Solid Edge part; units mm, degrees
sketch "Sketch1" plane through (0, 0, 0) normal (0, -1, 0) x (1, 0, 0)
  line L0 (-11.4484, 120) -> (-32.1539, 120)
  line L1 (-32.1539, 120) -> (0, 0)
  line L2 (0, 0) -> (20.7055, 0)
  line L3 (20.7055, 0) -> (-11.4484, 120)
extrude "Protrusion1" add sketch "Sketch1" against normal blind 20
hole "Agujero_3" at (-22.1539, 10, 120) direction (0, 0, -1) diameter 4.917 depth 24 tip angle 118 thread major 6 thread length 20
hole "Agujero_4" at (10.7055, 10, 0) direction (0, 0, 1) diameter 4.917 depth 24 tip angle 118 thread major 6 thread length 20
properties part number "1976-1100-002" material "Acero, estructural"
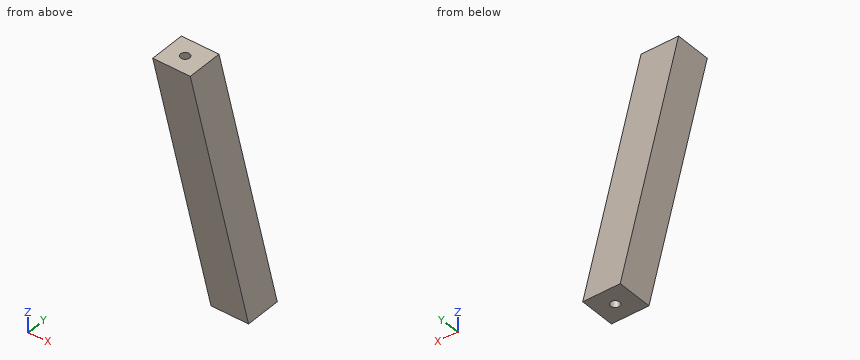
Read the model definition and answer for the solid it produces. Units are mm, in the model's axes. Coordinates: 2 decimals unless noted, no trailing zeros. Order: outer loops, then holes, each group sorted by start corner. A loop starts at its lowest first (then second) coordinate and runs counter-clockwise, first axis right, second up. Notation, with made-up numbers: M 24,-19.75 L 50,-19.75 A34 cw 50,18.25 Z; hole C 27,4.25 d2. An arc over 180 degrees is marked long. Put each result on its own line as item: value. Start each with the question number.
Item 1: Section C-C, the plane x = -18.5 is taken. Determine the outline of the cut face in (y, z), plus the area to 3 significant figures.
Item 2: Consider probe 1 along X at (y, z) = (10, 115); probe 2 along X at (y, z) = (10, 110.5); probe 3 along Y at (x, z) = (11.5, 6). Determine where each line is inside the solid, lowest interval first. Write a range as [from, to].
Item 3: Section A-A, the plane z = 16 is taken. Determine the outline of the cut face in (x, y).
Item 4: Given pin 1 Ø10 at (x, y) = (-4.5, 9) entering from -Z; pin 2 Ø2 at (y, z) = (16, 30.5) entering from -X; pin 3 Ø5 at (y, z) = (13, 51.5) entering from +X; pin 4 Ø1.5 at (y, z) = (7.5, 76.5) entering from +X, each flat-ended and moving along its own axis, determine where each tip first touches the part or whether it passes through.
Item 5: Section B-B, the plane y = 4.5 is taken. Determine the outline of the cut face in (x, z), plus the area to 3 significant figures.
Computed:
1. outline: M 0,69.04 L 20,69.04 L 20,120 L 0,120 Z
1. area: 1,020 mm2
2. probe 1: x = [-30.81, -24.61], [-19.7, -10.11]
2. probe 2: x = [-29.61, -24.61], [-19.7, -8.9]
2. probe 3: y = [0, 7.67], [12.33, 20]
3. outline: M -4.29,0 L 16.42,0 L 16.42,20 L -4.29,20 Z; hole C 10.71,10 d4.92
4. pin 1: stops at z = 0
4. pin 2: stops at x = -8.44
4. pin 3: stops at x = 7.58
4. pin 4: stops at x = 0.41
5. outline: M -32.15,120 L 0,0 L 20.71,0 L -11.45,120 Z
5. area: 2,480 mm2
